Design review of the part built by this model. Coordinates are the model's own, in mm. Face numbers are marked on the shaded views. Coordinates: 2 decimals unless noted, no trailing zeros. Write each loop counter-clockwise with the first axis right and the second up, starting at its lowest first coordinate (ties: lowest second). Pieces come first, ordered by that corner, then holes.
Q1. For L1, parallel to Y at x = -113.8, z = -8.5; L2, parallel to Y at x = 38, z = 57; L3, parallel to Y at x = -113, z = 8, list the stretches that pass through material, from the lowest coordinate up.
Q2. For pin 1 Ø6.5 at (y, z) = (25, 0) entering from +X; pin 2 Ø12 at (x, y) = (-43, 7.5) entering from -Z; pin 3 Ø12 at (y, z) = (20, -3.5) entering from +X; pin 4 Ø2 at (x, y) = (54.5, 6.5) entering from -Z, all flat-tipped, find the tip position at first contact; note any pin that passes through.
Q3. Take a section at C-C, the plane z = 53. Write out the cut boundary in (x, y), plus the area to 3 significant figures.
Q4. Take a section at B-B, the plane x = -77. Write out the cut boundary in (y, z), plus the area to 3 significant figures.
Q5. The part is to be moulded in two halves that separate along Z. For the marked faces 1, 2, 3 and 4, say which applies: released by +Z, released by -Z, zero draft, split by the parting line, or undercut.
Q6. Take a section at A-A, the plane y = 33. Write out the cut boundary in (x, z), plus the area to 3 significant figures.
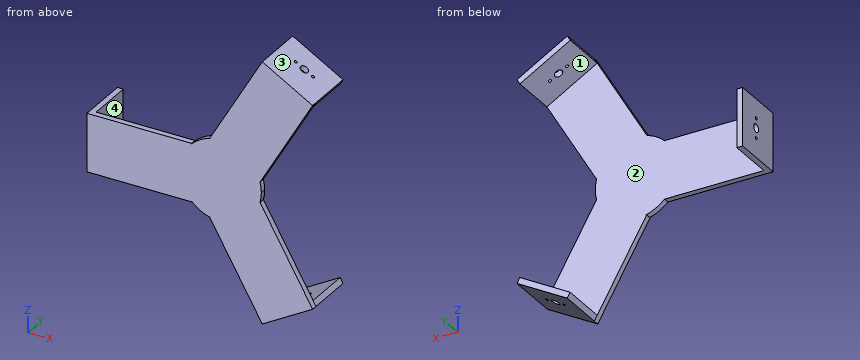
from build123d import *

# Parameters (mm, degrees)
ESQUISSE3_R             = 35
BOSS_EXTRU_3_DEPTH      = 5
ESQUISSE4_W             = 5
ESQUISSE4_H             = 50
BOSS_EXTRU_4_DEPTH      = 40
ESQUISSE5_R             = 3.5
ESQUISSE5_R_2           = 1.25
ENL_V_MAT_EXTRU_1_DEPTH = 225.427684996
ESQUISSE6_R             = 3.5
ESQUISSE6_R_2           = 1.25
ENL_V_MAT_EXTRU_2_DEPTH = 272.884889055
ESQUISSE7_R             = 3.5
ESQUISSE7_R_2           = 1.25
ENL_V_MAT_EXTRU_3_DEPTH = 272.884889055


with BuildPart() as part:
    # Esquisse3 → Boss.-Extru.3 (new body)
    with BuildSketch(Plane(origin=(0, 0, 0), x_dir=(1, 0, 0), z_dir=(0, 1, 0))):
        with BuildLine():
            Line((-115, -25), (-25, -25))
            Line((-25, -25), (-24.99494949, -24.500051021))
            ThreePointArc((-24.99494949, -24.500051021), (-34.998214236, 0.353553761), (-24.494897428, 25))
            Line((-24.494897428, 25), (-25, 25))
            Line((-25, 25), (-115, 25))
            Line((-115, 25), (-115, -25))
        make_face()
        Circle(ESQUISSE3_R)
        Polygon((-9.403186381, -33.713203436), (35.849364905, -112.092921435), (79.150635095, -87.092921435), (34.150635095, -9.150635095), align=None)
        with BuildLine():
            Line((-24.494897428, 25), (-24.99494949, -24.500051021))
            ThreePointArc((-24.99494949, -24.500051021), (-17.805293657, -30.132565736), (-9.403186381, -33.713203436))
            Line((-9.403186381, -33.713203436), (33.715141323, -9.396235714))
            ThreePointArc((33.715141323, -9.396235714), (34.677297662, -4.741837919), (35, 0))
            ThreePointArc((35, 0), (34.72342821, 4.391302011), (33.898083809, 8.713203436))
            Line((33.898083809, 8.713203436), (-8.720191833, 33.896286735))
            ThreePointArc((-8.720191833, 33.896286735), (-17.19292058, 30.486119496), (-24.494897428, 25))
        make_face()
        Circle(ESQUISSE3_R)
        Polygon((33.898083809, 8.713203436), (79.150635095, 87.092921435), (35.849364905, 112.092921435), (-9.150635095, 34.150635095), align=None)
        with BuildLine():
            ThreePointArc((33.898083809, 8.713203436), (17.805293657, 30.132565736), (-8.720191833, 33.896286735))
            Line((-8.720191833, 33.896286735), (33.898083809, 8.713203436))
        make_face()
    extrude(amount=BOSS_EXTRU_3_DEPTH)

    # Esquisse4 → Boss.-Extru.4 (add)
    with BuildSketch(Plane(origin=(0, 5, 0), x_dir=(1, 0, 0), z_dir=(0, 1, 0))):
        with Locations((-112.5, 0)):
            Rectangle(ESQUISSE4_W, ESQUISSE4_H)
        Polygon((35.849364905, 112.092921435), (79.150635095, 87.092921435), (76.650635095, 82.762794416), (33.349364905, 107.762794416), align=None)
        Polygon((79.150635095, -87.092921435), (76.650635095, -82.762794416), (33.349364905, -107.762794416), (35.849364905, -112.092921435), align=None)
    extrude(amount=BOSS_EXTRU_4_DEPTH)

    # Esquisse5 → Enl_v. mat.-Extru.1 (cut, through all)
    with BuildSketch(Plane(origin=(-110, 0, 0), x_dir=(0, 0, -1), z_dir=(1, 0, 0))):
        with Locations((0, 25)):
            Circle(ESQUISSE5_R)
        with Locations((-8.5, 25)):
            Circle(ESQUISSE5_R_2)
        with Locations((8.5, 25)):
            Circle(ESQUISSE5_R_2)
    extrude(amount=-ENL_V_MAT_EXTRU_1_DEPTH, mode=Mode.SUBTRACT)

    # Esquisse6 → Enl_v. mat.-Extru.2 (cut, through all)
    with BuildSketch(Plane(origin=(55, 0, 95.262794416), x_dir=(-0.8660254037844386, 0, 0.4999999999999999), z_dir=(-0.49999999999999994, 0, -0.8660254037844387))):
        with Locations((0, 25)):
            Circle(ESQUISSE6_R)
        with Locations((-8.5, 25)):
            Circle(ESQUISSE6_R_2)
        with Locations((8.5, 25)):
            Circle(ESQUISSE6_R_2)
    extrude(amount=-ENL_V_MAT_EXTRU_2_DEPTH, mode=Mode.SUBTRACT)

    # Esquisse7 → Enl_v. mat.-Extru.3 (cut, through all)
    with BuildSketch(Plane(origin=(55, 0, -95.262794416), x_dir=(0.8660254037844388, 0, 0.49999999999999983), z_dir=(-0.4999999999999998, 0, 0.8660254037844387))):
        with Locations((0, 25)):
            Circle(ESQUISSE7_R)
        with Locations((8.5, 25)):
            Circle(ESQUISSE7_R_2)
        with Locations((-8.5, 25)):
            Circle(ESQUISSE7_R_2)
    extrude(amount=-ENL_V_MAT_EXTRU_3_DEPTH, mode=Mode.SUBTRACT)


solid = part.part
Responses:
1. L1: y = 0 to 23.75, 26.25 to 45
1. L2: y = 0 to 5
1. L3: y = 0 to 23.85, 26.15 to 45
2. pin 1: passes through
2. pin 2: stops at z = -25
2. pin 3: stops at x = -110
2. pin 4: stops at z = -101.9
3. outline: (1.73, 0) - (59.47, 0) - (59.47, 5) - (1.73, 5) - close
3. area: 289 mm2
4. outline: (0, -25) - (5, -25) - (5, 25) - (0, 25) - close
4. area: 250 mm2
5. face 1: undercut
5. face 2: undercut
5. face 3: released by +Z
5. face 4: zero draft
6. outline: (-115, -25) - (-110, -25) - (-110, 25) - (-115, 25) - close; (33.35, -107.76) - (35.85, -112.09) - (79.15, -87.09) - (76.65, -82.76) - close; (33.35, 107.76) - (76.65, 82.76) - (79.15, 87.09) - (35.85, 112.09) - close
6. area: 750 mm2
